Check sheet for the drawn part. Datum: minimum x, y, z corner. Units: mm. A direction names the side the tool comes from. Coordinates: 2 decimals unless noted, no trailing zeros. Loops run counter-clockwise (first coordinate to the right, second up) from the corner with the lowest first, then second, coordinate; pieces in that order, holes last. Notation, with made-up numbers: M 23.25,22 L 54.25,22 A25 ccw 54.25,37 Z; hole C 75,-17 d3. An arc over 180 degrees is marked long. Answer in a Markdown table with one row per item. Add a question column.
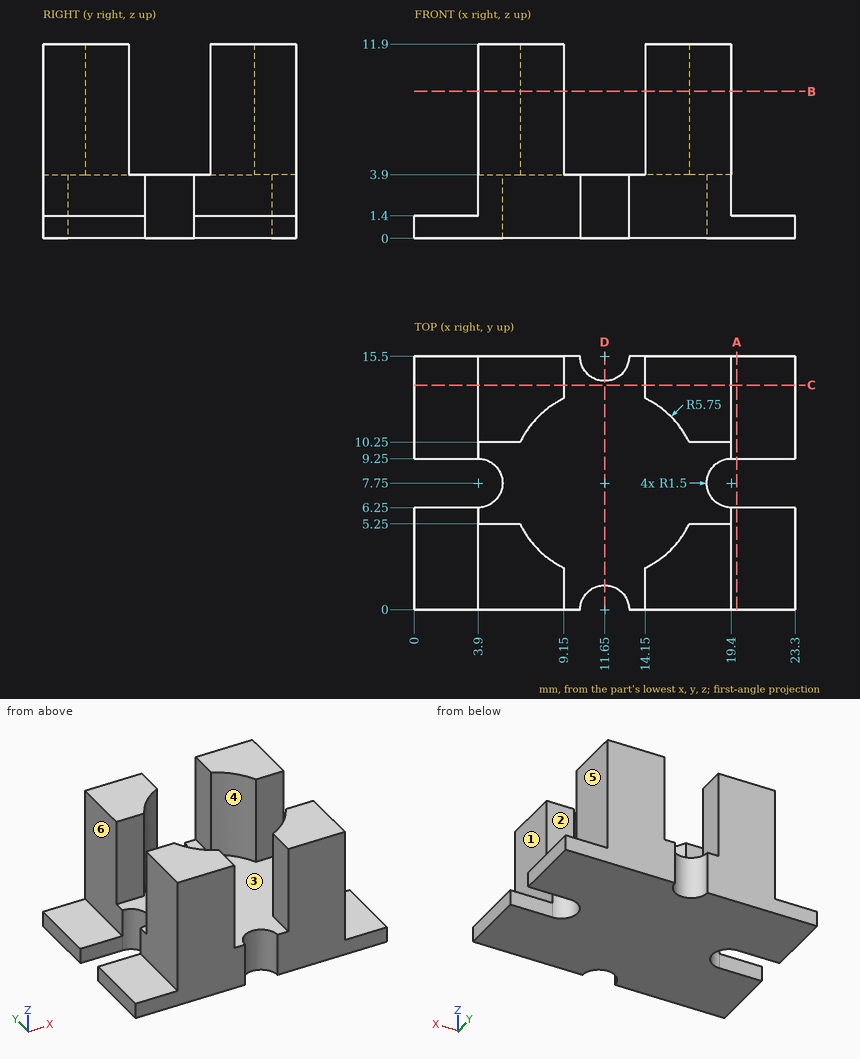
Q1. Cross-section at D-D (x = 11.65). Record the cut outline in (y, z), plus the area to 4 significant figures.
Q2. Access from +Z, -Z, +X, -X, +Y, -Y to the whole of each face (thin tool, end or side, straight path). Record for the marked faces 4, 5 and 6.
Q3. Thickness scan on L1, parallel to Y at x = 5, z = 5.5; L2, parallel to X at y = 12.75, z = 2.25; L3, parallel to Z at x = 14.5, y = 6.5. Record the ranges inside material, lowest first.
Q4. Cross-section at A-A (x = 19.75). Record the cut outline in (y, z), plus the area to 3 significant figures.
Q5. Cross-section at B-B (z = 9). Record the cut outline in (x, y), plus the area to 3 significant figures.
Q6. Mould release check, pull along X, two halves, no side actions. Record for the marked faces 1, 2 and 3: released by +X, released by -X, zero draft, split by the parting line, or undercut.
Q7. Cross-section at C-C (y = 13.75). Record the cut outline in (x, z), plus the area to 3 significant figures.
Q8. Go/stop test with flat-tipped pins: pin 1 (1.9 mm diameter, centred on y = 4, z = 7, fed in from +X); pin 2 (1.9 mm diameter, centred on y = 1.5, z = 9, fed in from -X); pin 3 (1.2 mm diameter, centred on x = 21.5, y = 13.5, fed in from +Z). Record where each tip stops, or that it passes through.
Answer key:
| question | item | result |
|---|---|---|
| 1 | outline | M 1.5,0 L 14,0 L 14,3.9 L 1.5,3.9 Z |
| 1 | area | 48.75 mm^2 |
| 2 | face 4 | +Z |
| 2 | face 5 | +Z, +X, +Y, -Y |
| 2 | face 6 | +Z, -X, +Y, -Y |
| 3 | L1 | 0 to 5.25, 10.25 to 15.5 |
| 3 | L2 | 3.9 to 19.4 |
| 3 | L3 | 0 to 3.9 |
| 4 | outline | M 0,0 L 6.25,0 L 6.25,1.4 L 0,1.4 Z; M 9.25,0 L 15.5,0 L 15.5,1.4 L 9.25,1.4 Z |
| 4 | area | 17.5 mm^2 |
| 5 | outline | M 3.9,0 L 9.15,0 L 9.15,2.57 A5.75 cw 6.47,5.25 L 3.9,5.25 Z; M 3.9,10.25 L 6.47,10.25 A5.75 cw 9.15,12.93 L 9.15,15.5 L 3.9,15.5 Z; M 14.15,0 L 19.4,0 L 19.4,5.25 L 16.83,5.25 A5.75 cw 14.15,2.57 Z; M 14.15,12.93 A5.75 cw 16.83,10.25 L 19.4,10.25 L 19.4,15.5 L 14.15,15.5 Z |
| 5 | area | 92.6 mm^2 |
| 6 | face 1 | released by +X |
| 6 | face 2 | zero draft |
| 6 | face 3 | undercut |
| 7 | outline | M 0,0 L 23.3,0 L 23.3,1.4 L 19.4,1.4 L 19.4,11.9 L 14.15,11.9 L 14.15,3.9 L 9.15,3.9 L 9.15,11.9 L 3.9,11.9 L 3.9,1.4 L 0,1.4 Z |
| 7 | area | 155 mm^2 |
| 8 | pin 1 | x = 19.4 |
| 8 | pin 2 | x = 3.9 |
| 8 | pin 3 | z = 1.4 |
